Read the model definition and answer for the solid it produces. Units are mm, in the model's axes. A direction names the side the tool comes from. Round coordinates to 2 decimals unless told otherwise and drop trailing zeros. Write each loop counter-clockwise with the first axis right and the second up, starting at its lowest first coordinate (ties: lowest second). Pieces come first, ordered by that corner, then holes. Notation, with made-up numbers: (-9.75, -15) -> (6.25, -15) arc R24 ccw to (6.25, 5) -> close; hole circle Ø9 at (35, 22). An arc over 180 degrees is marked (long way). Return JSON: item names as keys, results as strings. Group by question number.
(1) For faces 5 (the flat face through (70, 15, 100)), 6 (the cylindrical face through (39.223, 10.14, 59.96)), 7 (the flat face through (16, 5, 8)), 8 (the flat face through (85, 10, 100)), determine the directions among +Z, -Z, +X, -X, +Y, -Y from which every point of the face is accessible in a straight line to the end or side of a thin tool.
(2) A cutting plane is placed at C-C on z = 101.75. Give the vertices of the cut face in (x, y), then the cut area to 3 significant figures.
(3) The mould has two halves that part along Z. Classify faces 1 (the flat face through (49, 10, 0)), 2 (the cylindrical face through (63.223, 10.14, 59.96)), 3 (the flat face through (85, 15, 120)), 4 (the cylindrical face through (83.46, 14.93, 107.87)): released by +Z, released by -Z, zero draft, split by the parting line, or undercut.
(4) Straight lines are drawn through the part: line 1 (Z direction, x = 10, y = 14.25); line 2 (X direction, y = 13, z = 57.83); line 3 (Z direction, x = 81.75, y = 16.75). For each, find the intervals that lie inside material, in ascending order.
(5) A cutting plane is placed at A-A on x = 81.75. Give the vertices of the cut face in (y, z).
(6) A cutting plane is placed at D-D on y = 16. Give the vertices of the cut face in (x, z).
(7) A cutting plane is placed at B-B on y = 7. Give the vertices of the cut face in (x, z), then the cut area to 3 significant figures.
(8) Given pin 1 (6 mm diameter, centred on y = 17, z = 107, fed in from -X); pin 2 (13 mm diameter, centred on x = 4.5, z = 8, fed in from -Y); pin 3 (3 mm diameter, centred on x = 27.5, y = 12, fed in from +Z); pin 4 (2 mm diameter, centred on x = 10, z = 65, fed in from +Y), each flat-ended and moving along its own axis, determine where each tip first touches the part or whether it passes through.
Autodesk Inventor part; units mm, degrees
ref_plane "YZ Plane" through (0, 0, 0) normal (1, 0, 0) x (0, 1, 0)
ref_plane "XZ Plane" through (0, 0, 0) normal (0, 1, 0) x (-1, 0, 0)
ref_plane "XY Plane" through (0, 0, 0) normal (0, 0, 1) x (1, 0, 0)
sketch "Boceto1" plane through (0, 0, 0) normal (0, 1, 0) x (-1, 0, 0)
  line L0 (100, 80) -> (-100, 80)
  line L1 (-100, 80) -> (-100, -80)
  line L2 (-100, -80) -> (100, -80)
  line L3 (100, -80) -> (100, 80)
  line L4 (100, 80) -> (-100, -80) construction
  line L5 (-100, 80) -> (100, -80) construction
  point P0 (0, 0)
  dimension "d0" = 200
  dimension "d1" = 160
extrude "Extrusión1" add sketch "Boceto1" along normal blind 20
sketch "Boceto2" plane through (0, 20, 0) normal (0, 1, 0) x (1, 0, 0)
  circle A0 centre (-90, -57.83) radius 3.5
  line L0 (-100, -65.43) -> (-32, -65.43)
  line L1 (-32, -65.43) -> (-32, 14.57)
  line L2 (-32, 14.57) -> (-100, 14.57)
  line L3 (-100, 14.57) -> (-100, -65.43)
  line L4 (-66, -65.43) -> (-66, -8.508)
  circle A1 centre (-66, -57.83) radius 3.5
  circle A2 centre (-42, -57.83) radius 3.5
  line L5 (-32, -25.43) -> (-48.2072, -25.43)
  circle A3 centre (-42, 6.97) radius 3.5
  circle A4 centre (-66, 6.97) radius 3.5
  circle A5 centre (-90, 6.97) radius 3.5
  circle A6 centre (-60, 55) radius 5
  line L6 (-100, 80) -> (-100, -80)
  line L7 (0, 0) -> (0, -20.5185)
  circle A7 centre (90, -57.83) radius 3.5
  circle A8 centre (66, -57.83) radius 3.5
  circle A9 centre (42, -57.83) radius 3.5
  line L8 (100, -65.43) -> (32, -65.43)
  line L9 (66, -65.43) -> (66, -8.508)
  line L10 (32, -25.43) -> (48.2072, -25.43)
  circle A10 centre (90, 6.97) radius 3.5
  line L11 (100, 14.57) -> (100, -65.43)
  circle A11 centre (66, 6.97) radius 3.5
  line L12 (32, 14.57) -> (100, 14.57)
  line L13 (32, -65.43) -> (32, 14.57)
  circle A12 centre (42, 6.97) radius 3.5
  circle A13 centre (60, 55) radius 5
  line L14 (100, 80) -> (100, -80)
  dimension "d4" = 7
  dimension "d5" = 68
  dimension "d6" = 80
  dimension "d7" = 7.6
  dimension "d8" = 10
  dimension "d9" = 7
  dimension "d10" = 24
  dimension "d11" = 10
  dimension "d16" = 0
  dimension "d19" = 40
extrude "Extrusión2" cut sketch "Boceto2" against normal blind 20 contours A0 | A1 L4 | L4 A1 | A2 | A3 | A4 | A5 | A7 | A8 L9 | L9 A8 | A9 | A10 | A11 | A12
sketch "Boceto3" plane through (-100, 0, 80) normal (0, 0, 1) x (1, 0, 0)
  line L0 (0, 20) -> (30, 20)
  line L1 (30, 20) -> (30, 10)
  line L2 (30, 10) -> (0, 10)
  line L3 (0, 10) -> (0, 20)
  line L4 (100, 0) -> (100, 11.6249)
  line L5 (200, 20) -> (170, 20)
  line L6 (170, 20) -> (170, 10)
  line L7 (170, 10) -> (200, 10)
  line L8 (200, 10) -> (200, 20)
  dimension "d22" = 30
  dimension "d23" = 10
extrude "Extrusión3" add sketch "Boceto3" along normal blind 40
sketch "Boceto4" plane through (0, 20, 0) normal (0, 1, 0) x (1, 0, 0)
  line L0 (-60, 60) -> (-60, 50)
  line L1 (-70, 50) -> (-70, 60)
  line L2 (-60, 50) -> (-70, 60) construction
  line L3 (-70, 50) -> (-60, 60) construction
  line L4 (-60, 50) -> (-70, 50)
  circle A0 centre (-68.25, 51.75) radius 1.75
  line L5 (-70, 60) -> (-60, 60)
  circle A1 centre (-61.75, 58.25) radius 1.75
  line L6 (100, 80) -> (-100, 80)
  line L7 (0, 80) -> (0, 60)
  line L8 (60, 60) -> (60, 50)
  circle A2 centre (61.75, 58.25) radius 1.75
  line L9 (70, 60) -> (60, 60)
  line L10 (70, 50) -> (70, 60)
  line L11 (60, 50) -> (70, 60) construction
  line L12 (70, 50) -> (60, 60) construction
  line L13 (60, 50) -> (70, 50)
  circle A3 centre (68.25, 51.75) radius 1.75
  line L14 (-100, 80) -> (-100, -120)
  line L15 (100, 80) -> (100, -120)
  point P0 (0, 0)
  point P1 (-70.0286, 64.971)
  point P2 (-65, 50)
  point P3 (70.0286, 64.971)
  point P4 (65, 50)
  dimension "d26" = 1.75
  dimension "d27" = 8.25
  dimension "d28" = 20
  dimension "d29" = 10
  dimension "d30" = 10
  dimension "d31" = 1.75
  dimension "d32" = 1.75
  dimension "d33" = 1.75
  dimension "d58" = 30
  dimension "d59" = 30
extrude "Extrusión4" cut sketch "Boceto4" against normal blind 40 contours A1 | A0 | A2 | A3
sketch "Boceto5" plane through (0, 20, 0) normal (0, 1, 0) x (1, 0, 0)
  line L0 (-100, -80) -> (-100, -120)
  line L1 (-70.0001, -120) -> (-70.0001, -80)
  line L2 (-55.1959, -79.9497) -> (-70.0001, -80)
  line L3 (-70.0001, -80) -> (-100, -80)
  line L4 (-100, -120) -> (-70.0001, -120)
  line L5 (-64.3507, -80) -> (-74.3507, -80)
  circle A0 centre (-81.75, -108.25) radius 1.75
  circle A1 centre (-88.25, -101.75) radius 1.75
  line L6 (-70.0001, -80) -> (70.0001, -80)
  line L7 (0, -80) -> (0, -101.75)
  circle A2 centre (81.75, -108.25) radius 1.75
  circle A3 centre (88.25, -101.75) radius 1.75
  line L8 (-70, -80) -> (70, -80)
  line L9 (-100, 80) -> (-100, -120)
  point P0 (0, 0)
  point P1 (-81.75, -101.75)
  point P2 (-63.4459, -118.25)
  point P3 (81.75, -101.75)
  dimension "d36" = 11.7499
  dimension "d37" = 40
  dimension "d38" = 29.9999
  dimension "d39" = 21.75
  dimension "d40" = 11.75
  dimension "d41" = 28.3003
  dimension "d42" = 11.7499
  dimension "d43" = 0
  dimension "d44" = 0
hole "Agujero1" at (-88.25, 20, 101.75) at (-81.75, 20, 108.25) at (81.75, 20, 108.25) at (88.25, 20, 101.75) direction (0, -1, 0) diameter 3.5 end through all
ref_plane "Plano de trabajo1" through (100, 0, 0) normal (0, 0, -1) x (-1, 0, 0)
ref_plane "Plano de trabajo2" through (0, 0, -80) normal (-1, 0, 0) x (0, 0, 1)
sketch "Boceto6" plane through (0, 0, 0) normal (0, -1, 0) x (1, 0, 0)
  circle A0 centre (10, -10) radius 1.75
  line L0 (6.803, 0) -> (14.6069, 0)
  line L1 (0, 0) -> (0, -4.8284)
  line L2 (0, 0) -> (20.0354, 0)
  circle A1 centre (10, 10) radius 1.75
  line L3 (0, 0) -> (0, 4.8284)
  circle A2 centre (-10, 10) radius 1.75
  circle A3 centre (-10, -10) radius 1.75
  dimension "d63" = 3.5
  dimension "d64" = 10
  dimension "d65" = 10
hole "Agujero2" at (10, 0, 10) at (-10, 0, 10) at (-10, 0, -10) at (10, 0, -10) direction (0, 1, 0) diameter 3.5 end through all
sketch "Boceto7" plane through (0, 0, 0) normal (0, -1, 0) x (1, 0, 0)
  line L0 (-16, 16) -> (16, 16)
  line L1 (16, 16) -> (16, -16)
  line L2 (16, -16) -> (-16, -16)
  line L3 (-16, -16) -> (-16, 16)
  line L4 (-16, 16) -> (16, -16) construction
  line L5 (16, 16) -> (-16, -16) construction
  point P0 (0, 0)
  point P1 (0, 0)
  point P2 (0, 0)
  dimension "d73" = 32
  dimension "d74" = 32
extrude "Extrusión5" cut sketch "Boceto7" against normal blind 10
sketch "Boceto8" plane through (0, 20, 0) normal (0, 1, 0) x (1, 0, 0)
  line L0 (-15, -60) -> (15, -60)
  circle A0 centre (10, -65) radius 1.75
  line L1 (-10, -65) -> (10, -65)
  line L2 (15, -60) -> (15, -70)
  circle A1 centre (-10, -65) radius 1.75
  line L3 (-15, -70) -> (15, -60) construction
  line L4 (-15, -60) -> (15, -70) construction
  line L5 (-15, -70) -> (-15, -60)
  line L6 (15, -70) -> (-15, -70)
  point P0 (0, 0)
  point P1 (0, -69.1269)
  point P2 (-15, -67.1661)
  point P3 (0, -69.1269)
  point P4 (15, -65)
  dimension "d77" = 10
  dimension "d78" = 30
  dimension "d79" = 5
  dimension "d80" = 5
  dimension "d81" = 5
  dimension "d82" = 5
hole "Agujero3" at (-10, 20, 65) at (10, 20, 65) direction (0, -1, 0) diameter 3.5 end through all
split "Dividir1" plane through (100, 0, 0) removes the side toward (0, 0, -1)
split "Dividir2" plane through (0, 0, -80) removes the side toward (-1, 0, 0)
properties part number "base_back_4"
Checks:
{
 "1": {"face 5": "+Z, -X, +Y, -Y", "face 6": "+Y, -Y", "face 7": "-Z, -X, -Y", "face 8": "+Z, +X, -X, -Y"},
 "2": {"outline": "(70, 10) -> (86.5, 10) -> (86.5, 20) -> (70, 20) -> close; (90, 10) -> (100, 10) -> (100, 20) -> (90, 20) -> close", "area": "265 mm^2"},
 "3": {"face 1": "released by -Z", "face 2": "undercut", "face 3": "released by +Z", "face 4": "undercut"},
 "4": {"line 1": "z = 0 to 8.25, 11.75 to 63.25, 66.75 to 80", "line 2": "x = 0 to 38.5, 45.5 to 62.5, 69.5 to 86.5, 93.5 to 100", "line 3": "z = 0 to 106.5, 110 to 120"},
 "5": {"outline": "(0, 0) -> (20, 0) -> (20, 106.5) -> (10, 106.5) -> (10, 80) -> (0, 80) -> close; (10, 110) -> (20, 110) -> (20, 120) -> (10, 120) -> close"},
 "6": {"outline": "(0, 0) -> (100, 0) -> (100, 120) -> (70, 120) -> (70, 80) -> (0, 80) -> close; hole circle Ø3.5 at (10, 10); hole circle Ø3.5 at (10, 65); hole circle Ø7 at (42, 57.83); hole circle Ø7 at (66, 57.83); hole circle Ø3.5 at (81.75, 108.25); hole circle Ø7 at (90, 57.83); hole circle Ø3.5 at (88.25, 101.75)"},
 "7": {"outline": "(0, 16) -> (16, 16) -> (16, 0) -> (100, 0) -> (100, 80) -> (0, 80) -> close; hole circle Ø3.5 at (10, 65); hole circle Ø7 at (42, 57.83); hole circle Ø7 at (66, 57.83); hole circle Ø7 at (90, 57.83)", "area": "7,620 mm^2"},
 "8": {"pin 1": "stops at x = 70", "pin 2": "stops at y = 10", "pin 3": "stops at z = 80", "pin 4": "passes through"}
}
